Source: three-view drawing plus pictorial views. Frame: mm from the lowest corner of the part. A direction names the side the tool comes from. Round coordinates to 2 decimals unless told otherwise and drop trailing zeros. Loops run counter-clockwise (first coordinate to the right, second up) from the corner with the lowest first, then second, coordinate; pieces in that order, holes last. Notation, with made-up numbers: M 61.25,5 L 115.25,5 A24 ccw 115.25,15 Z; hole C 42.25,-5.75 d6. An arc over 180 degrees is marked long. Answer as a JSON object with one key per item and string values.
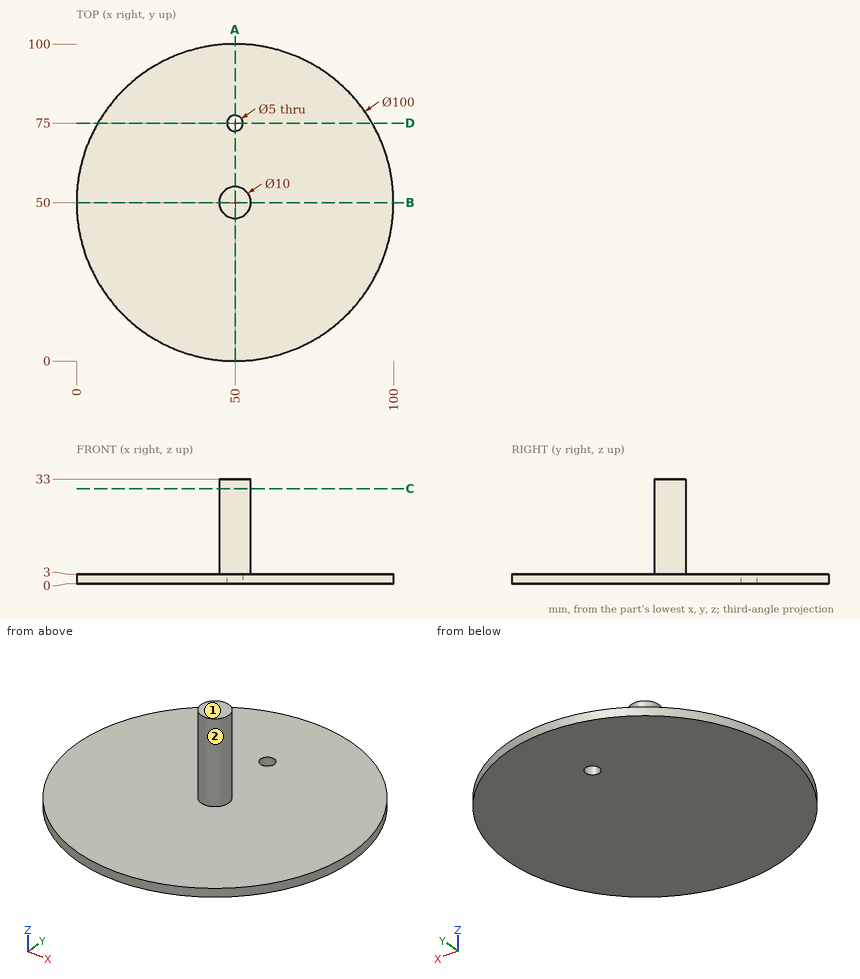
1) Cut plane C-C on z = 30. Return the cut outline in (x, y), and give its area (3 significant figures).
Geometry results:
{"outline": "C 50,50 d10", "area": "78.5 mm2"}
2) Cut plane D-D on y = 75. Return the cut outline in (x, z).
Geometry results:
{"outline": "M 6.7,0 L 47.5,0 L 47.5,3 L 6.7,3 Z; M 52.5,0 L 93.3,0 L 93.3,3 L 52.5,3 Z"}
3) Line query: probe 1 along Y at (x, z) = (50, 1.4); probe 2 along Z at (x, y) = (48, 29); probe 3 along X at (y, z) = (75, 2.4). Output: solid intervals per line, ascending.
Geometry results:
{"probe 1": "0 to 72.5, 77.5 to 100", "probe 2": "0 to 3", "probe 3": "6.7 to 47.5, 52.5 to 93.3"}
4) Cut plane B-B on y = 50. Return the cut outline in (x, z), and give its area (3 significant figures).
Geometry results:
{"outline": "M 0,0 L 100,0 L 100,3 L 55,3 L 55,33 L 45,33 L 45,3 L 0,3 Z", "area": "600 mm2"}
5) First-contact query: pin 1 (6 mm diameter, centred on x = 49, z = 13, fed in from -Y); pin 2 (12 mm diameter, centred on x = 53, z = 23.5, fed in from +Y); pin 3 (5 mm diameter, centred on x = 13.5, y = 77, fed in from -Z); pin 4 (12 mm diameter, centred on y = 19, z = 3.5, fed in from -X). Flat tips, straight axial feed; report the tip coordinate or a pass-through.
Geometry results:
{"pin 1": "y = 45", "pin 2": "y = 55", "pin 3": "z = 0", "pin 4": "x = 6.71"}
6) Set-up query: the marked faces 1 and 2. Return all of +Z, -Z, +X, -X, +Y, -Y with unobstructed straight access to the full face (end or side cutting, diameter ignored); none if empty.
Geometry results:
{"face 1": "+Z, +X, -X, +Y, -Y", "face 2": "+Z"}
7) Cut plane A-A on x = 50. Return the cut outline in (y, z).
Geometry results:
{"outline": "M 0,0 L 72.5,0 L 72.5,3 L 55,3 L 55,33 L 45,33 L 45,3 L 0,3 Z; M 77.5,0 L 100,0 L 100,3 L 77.5,3 Z"}
